Can you work these out from the model? Positions are in its coordinate system, mm. Face numbers are marked on the shaded views. A direction names the side the tool comes from. Coordinates: 2 decimals unless noted, no trailing zeros. Order: outer loops, then holes, each group sorted by start corner. A loop starts at its lowest first (then second) coordinate and runs counter-clockwise, first axis right, second up. Notation, with made-up numbers: M 14,-31.5 L 50,-31.5 A22 cw 50,-13.5 Z; hole C -3,52.25 d9. An arc over 180 degrees is marked long. Answer as a JSON object with one key per item and string values.
from build123d import *

# Parameters (mm, degrees)
F0_R     = 8.75
F1_DEPTH = 30
F3_DEPTH = 4.9
F5_D     = 5


with BuildPart() as f1:
    # F0 (on Top) → F1 (new body)
    with BuildSketch(Plane.XY):
        Circle(F0_R)
    extrude(amount=F1_DEPTH)

    # F2 (on face) → F3 (join)
    with BuildSketch(Plane.XY.offset(30)):
        with BuildLine():
            ThreePointArc((8.249579, 2.916667), (0, 8.75), (-8.249579, 2.916667))
            Line((-8.249579, 2.916667), (-12.15496, 2.916667))
            ThreePointArc((-12.15496, 2.916667), (-12.5, 0), (-12.15496, -2.916667))
            Line((-12.15496, -2.916667), (-8.249579, -2.916667))
            ThreePointArc((-8.249579, -2.916667), (0, -8.75), (8.249579, -2.916667))
            Line((8.249579, -2.916667), (12.15496, -2.916667))
            ThreePointArc((12.15496, -2.916667), (12.5, 0), (12.15496, 2.916667))
            Line((12.15496, 2.916667), (8.249579, 2.916667))
        make_face()
    extrude(amount=F3_DEPTH)

    # F5 (through all)
    with Locations(Plane(origin=(0, 0, 0), x_dir=(1, 0, 0), z_dir=(0, 0, -1))):
        with Locations((0, 0)):
            Hole(F5_D / 2)


solid = f1.part
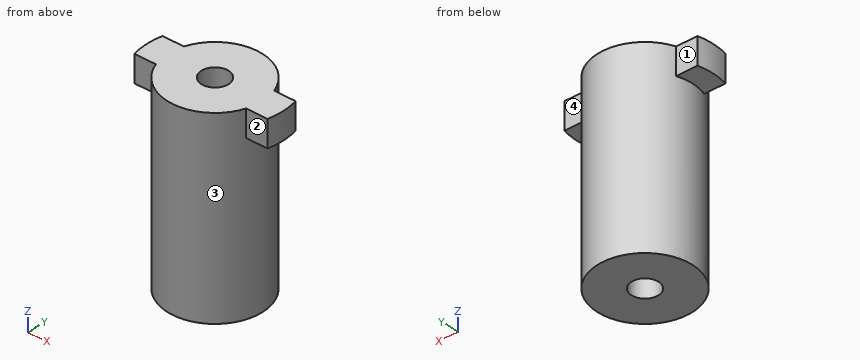
Item 1: I want a section at C-C, the plane z = 33.5. Write out the boundary of the cut face in (x, y).
Answers follow:
{"outline": "M -12.15,-2.92 L -8.25,-2.92 A8.75 ccw 8.25,-2.92 L 12.15,-2.92 A12.5 ccw 12.15,2.92 L 8.25,2.92 A8.75 ccw -8.25,2.92 L -12.15,2.92 A12.5 ccw Z; hole C 0,0 d5"}
Item 2: I want a section at D-D, the plane x = -9.75. Write out the boundary of the cut face in (y, z), plus the area to 3 significant figures.
Answers follow:
{"outline": "M -2.92,30 L 2.92,30 L 2.92,34.9 L -2.92,34.9 Z", "area": "28.6 mm^2"}
Item 3: I want a section at B-B, the plane x = 0. Write out the boundary of the cut face in (y, z), plus the area to 3 significant figures.
Answers follow:
{"outline": "M -8.75,0 L -2.5,0 L -2.5,34.9 L -8.75,34.9 Z; M 2.5,0 L 8.75,0 L 8.75,34.9 L 2.5,34.9 Z", "area": "436 mm^2"}
Item 4: Which directions (+Z, -Z, +X, -X, +Y, -Y) give clear straight access to the entire face, cutting with the end or side of a thin tool? Please do the marked faces 1, 2, 3 and 4.
Answers follow:
{"face 1": "+Z, -Z, -X, +Y", "face 2": "+Z, -Z, +X, -Y", "face 3": "-Z", "face 4": "+Z, -Z, +X, +Y"}
Item 5: I want a section at A-A, the plane y = 0. Write out the boundary of the cut face in (x, z), plus the area to 3 significant figures.
Answers follow:
{"outline": "M -12.5,30 L -8.75,30 L -8.75,0 L -2.5,0 L -2.5,34.9 L -12.5,34.9 Z; M 2.5,0 L 8.75,0 L 8.75,30 L 12.5,30 L 12.5,34.9 L 2.5,34.9 Z", "area": "473 mm^2"}
Item 6: I'm going to push flat-ended pins straight in: pin 1 (6 mm diameter, centred on x = -7.5, z = 29, fed in from +Y); pin 2 (5 mm diameter, centred on y = 2.5, z = 8.5, fed in from +X); pin 3 (3 mm diameter, centred on x = -10, z = 32.5, fed in from +Y). Where does each tip first touch, or does it pass through?
Answers follow:
{"pin 1": "stops at y = 7.5", "pin 2": "stops at x = 8.75", "pin 3": "stops at y = 2.92"}
Item 7: Please list where these lines run through material, in increasing order: line 1 (Y direction, x = 0, z = 12.5); line 2 (Y direction, x = 10, z = 30.5); line 3 (Z direction, x = 10, y = 0.25).
Answers follow:
{"line 1": "y = -8.75 to -2.5, 2.5 to 8.75", "line 2": "y = -2.92 to 2.92", "line 3": "z = 30 to 34.9"}
